Autodesk Inventor part; units mm, degrees
ref_plane "YZ Plane" through (0, 0, 0) normal (1, 0, 0) x (0, 1, 0)
ref_plane "XZ Plane" through (0, 0, 0) normal (0, 1, 0) x (-1, 0, 0)
ref_plane "XY Plane" through (0, 0, 0) normal (0, 0, 1) x (1, 0, 0)
sketch "Sketch1" plane through (0, 0, 0) normal (0, 0, 1) x (1, 0, 0)
  line L0 (-42.5, 28) -> (42.5, 28)
  line L1 (42.5, 28) -> (42.5, -28)
  line L2 (42.5, -28) -> (-42.5, -28)
  line L3 (-42.5, -28) -> (-42.5, 28)
  line L4 (-42.5, 28) -> (42.5, -28) construction
  line L5 (42.5, 28) -> (-42.5, -28) construction
  line L6 (-50, 35) -> (50, 35)
  line L7 (50, 35) -> (50, -35)
  line L8 (50, -35) -> (-50, -35)
  line L9 (-50, -35) -> (-50, 35)
  line L10 (-50, 35) -> (50, -35) construction
  line L11 (50, 35) -> (-50, -35) construction
  circle A0 centre (39, -24.5) radius 3.5
  circle A1 centre (39, 24.5) radius 3.5
  circle A2 centre (-19, 24.5) radius 3.5
  circle A3 centre (-19, -24.5) radius 3.5
  point P0 (0, 0)
  dimension "d0" = 85
  dimension "d1" = 56
  dimension "d2" = 100
  dimension "d3" = 70
  dimension "d4" = 7
  dimension "d5" = 7
  dimension "d6" = 3.5
  dimension "d7" = 3.5
  dimension "d8" = 3.5
  dimension "d9" = 3.5
  dimension "d10" = 7
  dimension "d11" = 7
  dimension "d12" = 58
  dimension "d13" = 58
  dimension "d14" = 3.5
  dimension "d15" = 3.5
extrude "Extrusion1" add sketch "Sketch1" along normal blind 4 contours L0 A1 L1 A0 L2 L3 | L0 L1 A1 | A0 L1 L2 | L6 L7 L8 L9
sketch "Sketch2" plane through (0, 0, 0) normal (0, 0, -1) x (-1, 0, 0)
  circle A0 centre (19, 24.5) radius 3.5
  circle A1 centre (19, 24.5) radius 3.5
  circle A2 centre (19, 24.5) radius 1.75
  circle A3 centre (-39, 24.5) radius 3.5
  circle A4 centre (-39, 24.5) radius 3.5
  circle A5 centre (-39, 24.5) radius 1.75
  circle A6 centre (-39, -24.5) radius 3.5
  circle A7 centre (-39, -24.5) radius 3.5
  circle A8 centre (-39, -24.5) radius 1.75
  circle A9 centre (19, -24.5) radius 3.5
  circle A10 centre (19, -24.5) radius 3.5
  circle A11 centre (19, -24.5) radius 1.75
  point P0 (0, 0)
  dimension "d18" = 3.5
  dimension "d19" = 3.5
  dimension "d20" = 3.5
  dimension "d21" = 3.5
extrude "Extrusion2" add sketch "Sketch2" against normal blind 10
sketch "Sketch3" plane through (0, 0, 0) normal (0, 0, -1) x (-1, 0, 0)
  line L0 (-38.5, 31.075) -> (-1.5, 31.075)
  line L1 (-1.5, 31.075) -> (-1.5, 8.925)
  line L2 (-1.5, 8.925) -> (-38.5, 8.925)
  line L3 (-38.5, 8.925) -> (-38.5, 31.075)
  line L4 (-38.5, 31.075) -> (-1.5, 8.925) construction
  line L5 (-1.5, 31.075) -> (-38.5, 8.925) construction
  line L6 (-50, 35) -> (-50, -35)
  line L7 (50, 35) -> (-50, 35)
  line L8 (-32.75, 28.75) -> (-7.25, 28.75)
  line L9 (-7.25, 28.75) -> (-7.25, 11.25)
  line L10 (-7.25, 11.25) -> (-32.75, 11.25)
  line L11 (-32.75, 11.25) -> (-32.75, 28.75)
  line L12 (-32.75, 28.75) -> (-7.25, 11.25) construction
  line L13 (-7.25, 28.75) -> (-32.75, 11.25) construction
  circle A0 centre (-32.75, 28.75) radius 3
  circle A1 centre (-7.25, 28.75) radius 3
  circle A2 centre (-7.25, 11.25) radius 3
  circle A3 centre (-32.75, 11.25) radius 3
  circle A4 centre (-32.75, 11.25) radius 1.75
  circle A5 centre (-32.75, 28.75) radius 1.75
  circle A6 centre (-7.25, 28.75) radius 1.75
  circle A7 centre (-7.25, 11.25) radius 1.75
  point P0 (0, 0)
  point P1 (-20, 20)
  dimension "d24" = 37
  dimension "d25" = 22.15
  dimension "d26" = 30
  dimension "d28" = 15
  dimension "d29" = 25.5
  dimension "d30" = 17.5
  dimension "d31" = 6
  dimension "d32" = 6
  dimension "d33" = 6
  dimension "d34" = 6
  dimension "d35" = 3.5
  dimension "d36" = 3.5
  dimension "d37" = 3.5
  dimension "d38" = 3.5
extrude "Extrusion3" add sketch "Sketch3" along normal blind 10 contours A0 L0 | L0 A0 L8 A5 L11 | L11 A5 L8 A0 | A3 L11 A4 L10 L2 | L2 A3 | A1 L0 | L0 A1 L9 A6 L8 | A3 L10 A4 L11 | L8 A6 L9 A1 | A2 L10 A7 L9 L2 | L2 A2 | A2 L9 A7 L10
sketch "Sketch5" plane through (0, 0, 0) normal (0, 0, -1) x (-1, 0, 0)
  line L0 (-36.5, -7.5) -> (6.5, -7.5)
  line L1 (6.5, -7.5) -> (6.5, -28.5)
  line L2 (6.5, -28.5) -> (-36.5, -28.5)
  line L3 (-36.5, -28.5) -> (-36.5, -7.5)
  line L4 (-36.5, -7.5) -> (6.5, -28.5) construction
  line L5 (6.5, -7.5) -> (-36.5, -28.5) construction
  line L6 (-50, -35) -> (50, -35)
  line L7 (-50, 35) -> (-50, -35)
  line L8 (-30.15, -9.85) -> (0.15, -9.85)
  line L9 (0.15, -9.85) -> (0.15, -26.15)
  line L10 (0.15, -26.15) -> (-30.15, -26.15)
  line L11 (-30.15, -26.15) -> (-30.15, -9.85)
  line L12 (-30.15, -9.85) -> (0.15, -26.15) construction
  line L13 (0.15, -9.85) -> (-30.15, -26.15) construction
  circle A0 centre (0.15, -9.85) radius 3
  circle A1 centre (-30.15, -9.85) radius 3
  circle A2 centre (-30.15, -26.15) radius 3
  circle A3 centre (0.15, -26.15) radius 3
  line L14 (20.5, -21.5) -> (20.5, 21.5)
  line L15 (20.5, 21.5) -> (41.5, 21.5)
  line L16 (41.5, 21.5) -> (41.5, -21.5)
  line L17 (41.5, -21.5) -> (20.5, -21.5)
  line L18 (20.5, -21.5) -> (41.5, 21.5) construction
  line L19 (20.5, 21.5) -> (41.5, -21.5) construction
  line L20 (22.85, -15.15) -> (22.85, 15.15)
  line L21 (22.85, 15.15) -> (39.15, 15.15)
  line L22 (39.15, 15.15) -> (39.15, -15.15)
  line L23 (39.15, -15.15) -> (22.85, -15.15)
  line L24 (22.85, -15.15) -> (39.15, 15.15) construction
  line L25 (22.85, 15.15) -> (39.15, -15.15) construction
  circle A4 centre (22.85, 15.15) radius 3
  circle A5 centre (22.85, -15.15) radius 3
  circle A6 centre (39.15, -15.15) radius 3
  circle A7 centre (39.15, 15.15) radius 3
  line L26 (50, -35) -> (50, 35)
  point P0 (0, 0)
  point P1 (-15, -18)
  point P2 (31, 0)
  dimension "d49" = 43
  dimension "d50" = 21
  dimension "d51" = 17
  dimension "d52" = 35
  dimension "d53" = 30.3
  dimension "d54" = 16.3
  dimension "d55" = 6
  dimension "d56" = 6
  dimension "d57" = 6
  dimension "d58" = 6
  dimension "d59" = 43
  dimension "d60" = 21
  dimension "d61" = 30.3
  dimension "d62" = 16.3
  dimension "d63" = 6
  dimension "d64" = 6
  dimension "d65" = 6
  dimension "d66" = 6
  dimension "d67" = 35
  dimension "d68" = 19
extrude "Extrusion4" add sketch "Sketch5" along normal blind 10 contours A1 L0 | L0 A1 L8 L11 | L11 L8 A1 | A2 L11 L10 L2 | L2 A2 | A0 L0 | L0 A0 L9 L8 | A2 L10 L11 | L8 L9 A0 | A3 L10 L9 L2 | L2 A3 | A3 L9 L10 | A5 L14 | L14 A5 L20 L23 | L23 L20 A5 | A6 L23 L22 L16 | L16 A6 | A4 L14 | L14 A4 L21 L20 | A6 L22 L23 | L20 L21 A4 | A7 L22 L21 L16 | L16 A7 | A7 L21 L22
sketch "Sketch6" plane through (32.75, 28.75, -10) normal (0, 0, -1) x (-1, 0, 0)
  circle A0 centre (0, 0) radius 1.75
  circle A1 centre (25.5, 0) radius 1.75
  circle A2 centre (25.5, -17.5) radius 1.75
  circle A3 centre (0, -17.5) radius 1.75
  circle A4 centre (2.6, -38.6) radius 3
  circle A5 centre (2.6, -54.9) radius 3
  circle A6 centre (32.9, -54.9) radius 3
  circle A7 centre (32.9, -38.6) radius 3
  circle A8 centre (55.6, -43.9) radius 3
  circle A9 centre (55.6, -13.6) radius 3
  circle A10 centre (71.9, -13.6) radius 3
  circle A11 centre (71.9, -43.9) radius 3
  point P0 (32.75, -28.75)
hole "Hole2" at (32.75, 28.75, -10) at (7.25, 28.75, -10) at (7.25, 11.25, -10) at (32.75, 11.25, -10) at (30.15, -9.85, -10) at (30.15, -26.15, -10) at (-0.15, -26.15, -10) at (-0.15, -9.85, -10) at (-22.85, -15.15, -10) at (-22.85, 15.15, -10) at (-39.15, 15.15, -10) at (-39.15, -15.15, -10) at (32.75, 28.75, -10) at (7.25, 28.75, -10) at (7.25, 11.25, -10) at (32.75, 11.25, -10) at (30.15, -9.85, -10) at (30.15, -26.15, -10) at (-0.15, -9.85, -10) at (-0.15, -26.15, -10) at (-22.85, -15.15, -10) at (-39.15, -15.15, -10) at (-39.15, 15.15, -10) at (-22.85, 15.15, -10) direction (0, 0, 1) diameter 3.5 end through all
chamfer "Chamfer1" distance 2 angle 45 15 edges at (35.75, 28.75, 0) (35.75, 11.25, 0) (10.25, 28.75, 0) (10.25, 11.25, 0) (-19.85, 15.15, 0) (2.85, -9.85, 0) (-19.85, -15.15, 0) (2.85, -26.15, 0) (33.15, -26.15, 0) (-36.15, 15.15, 0) (-36.15, -15.15, 0) (-15.5, -24.5, 4) (-15.5, 24.5, 4) (42.5, 24.5, 4) (42.5, -24.5, 4)
sketch "Sketch7" plane through (-50, 35, 0) normal (0, 1, 0) x (1, 0, 0)
  line L0 (-0.15, 13.5) -> (99.85, 13.5)
  line L1 (99.85, 13.5) -> (99.85, -16.5)
  line L2 (99.85, -16.5) -> (-0.15, -16.5)
  line L3 (-0.15, -16.5) -> (-0.15, 13.5)
  line L4 (-0.15, 13.5) -> (99.85, -16.5) construction
  line L5 (99.85, 13.5) -> (-0.15, -16.5) construction
  line L6 (0, 0) -> (100, 0)
  point P0 (50, 0)
  point P1 (49.85, -1.5)
  dimension "d81" = 100
  dimension "d82" = 30
  dimension "d83" = 1.5
extrude "Extrusion5" add sketch "Sketch7" along normal blind 4
sketch "Sketch8" plane through (-50, 35, 0) normal (0, -1, 0) x (1, 0, 0)
  line L0 (99.85, 16.5) -> (-0.15, 16.5)
  line L1 (99.85, 4) -> (99.85, 16.5)
  point P0 (50, 0)
  point P1 (66.5167, -6)
  point P2 (33.1833, -6)
  dimension "d86" = 22.5
  dimension "d87" = 22.5
  dimension "d88" = 33.3333
  dimension "d89" = 66.6667
hole "Hole3" at (16.5167, 35, -6) at (-16.8167, 35, -6) direction (0, 1, 0) diameter 5 end through all
equation "\"d4\" = d10"
equation "\"d5\" = d10"
equation "\"d11\" = d10"
equation "\"d13\" = d12"
properties part number "Eletronica - Raspberry"
Part model, mm, in its own coordinate system. A direction names the side the tool comes from. Round coordinates to 2 decimals unless told otherwise and drop trailing zeros. Order: outer loops, then holes, each group sorted by start corner. A loop starts at its lowest first (then second) coordinate and runs counter-clockwise, first axis right, second up. Notation, with made-up numbers: M 87.5,37 L 103.5,37 A16 cw 103.5,45 Z; hole C -31,2 d2. An arc over 180 degrees is marked long. Put each result on its own line as item: value. Start each with the question number.
1. Slice it at A-A on z = 2.5. State how many separate pieces and enclosed holes the cut face has, then the cut area to 3 significant figures.
2. Tool access for faces 1 (the face through (0.5, -23.22, -5.94)), 2 (the face through (-50, 0, 2)), 3 (the face through (-17, -25, 10)): list every direction of +Z, -Z, +X, -X, +Y, -Y with a clear straight run to the whole face (end or side of a thin tool).
3. Drill centre lines: probe 1 along X at (y, z) = (11.25, -4.75); probe 2 along X at (y, z) = (-10, -6.25); probe 3 along X at (y, z) = (-15.15, 0.75). Where is each one in solid material? Low to high. Write a range as [from, to].
4. Slice it at D-D on x = -11. List the corners of the cut face in (y, z), then the cut area to 3 significant figures.
5. Slice it at B-B on x = 39. List the corners of the cut face in (y, z).
6. Drop flat-ended pins along their axis: pin 1 (1.8 mm diameter, centred on x = -40, y = 14.5, fed in from -Z); pin 2 (12 mm diameter, centred on x = -40, y = 25.5, fed in from +Z); pin 3 (4 mm diameter, centred on y = 7, z = 3.5, fed in from -X). Give the stop position or say it passes through.
7. Two-plate mould, pull along Z, no slides. Class faces 4 (the face through (-15.86, 37.03, -8.31)), 5 (the face through (-1.885, -10.078, -2.902)), 6 (the face through (31, 27, -10)): +Z half, -Z half, draft (parallel to the pull), parting line (faces both ways), or undercut.
Findings:
1. separate pieces: 1
1. enclosed holes: 16
1. area: 7,250 mm2
2. face 1: -Z
2. face 2: +Z, -Z, -X, -Y
2. face 3: +Z, +X, -X, -Y
3. probe 1: [4.25, 5.5], [9, 10.25], [29.75, 31], [34.5, 35.75]
3. probe 2: [-3.15, -1.89], [1.59, 2.85], [27.15, 28.41], [31.89, 33.15]
3. probe 3: [-50, -40.9], [-37.4, -24.6], [-21.1, 50]
4. outline: M -35,0 L 35,0 L 35,-13.5 L 39,-13.5 L 39,16.5 L 35,16.5 L 35,4 L -35,4 Z
4. area: 400 mm2
5. outline: M -35,0 L -26.25,0 L -26.25,10 L -28,10 L -28,6 L -30,4 L -35,4 Z; M -22.75,0 L 22.75,0 L 22.75,10 L 21,10 L 21,6 L 19,4 L -19,4 L -21,6 L -21,10 L -22.75,10 Z; M 26.25,0 L 35,0 L 35,-13.5 L 39,-13.5 L 39,16.5 L 35,16.5 L 35,4 L 30,4 L 28,6 L 28,10 L 26.25,10 Z
6. pin 1: z = -10
6. pin 2: z = 4
6. pin 3: x = -50
7. face 4: undercut
7. face 5: draft
7. face 6: -Z half
